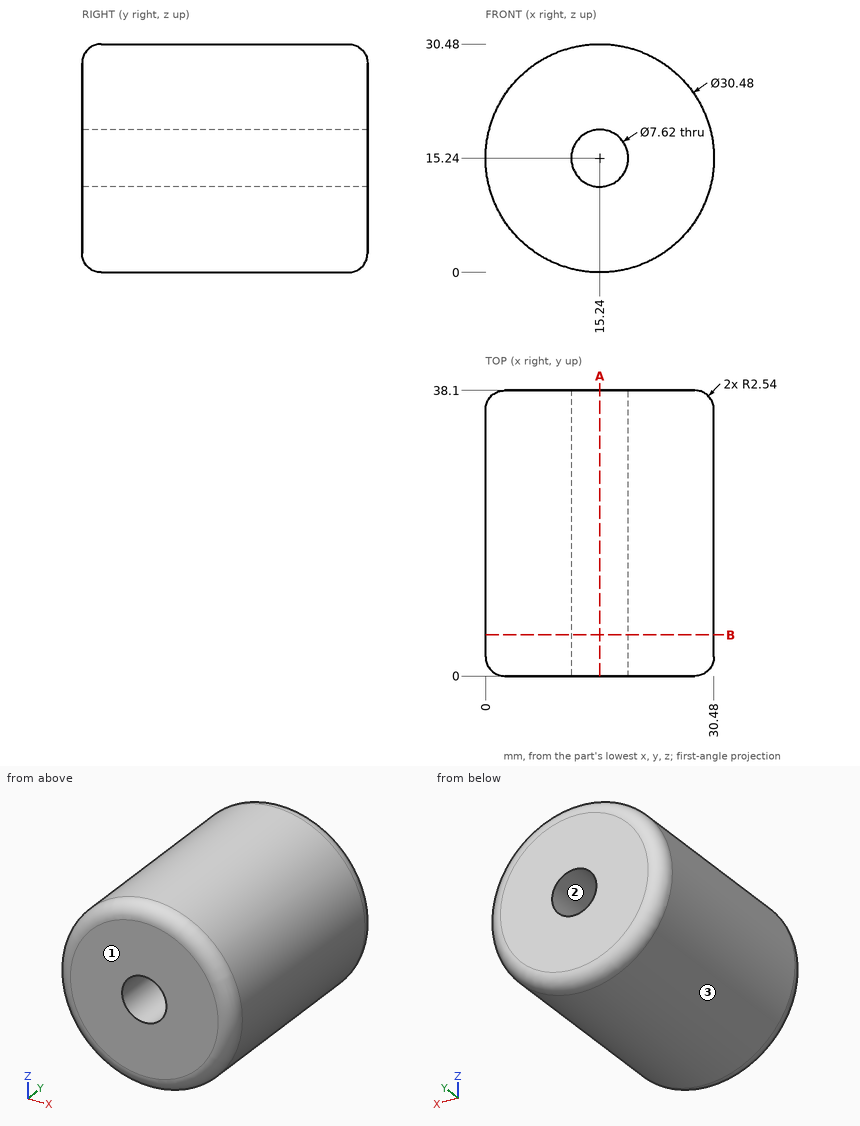
Source: three-view drawing plus pictorial views. Frame: mm from the lowest corner of the part. Give positions to 0.01 mm unless a question says otherwise; leave off trailing zeros. Loops run counter-clockwise (first coordinate to the right, second up) from the corner with the lowest first, then second, coordinate; pieces in that order, holes last. Notation, with made-up numbers: M -16,28 L 19,28 A34 cw 19,61 Z; hole C -27,-28.5 d8. An arc over 180 degrees is marked long. Use CSV: the item, a comma, the result in double quotes.
(1) Section B-B, the plane y = 5.5. Return loops of the section in (x, z).
Outcome:
outline,"C 15.24,15.24 d30.48; hole C 15.24,15.24 d7.62"
(2) Pull-direction query (X, two-part tool) for the marked faces 1, 2 and 3; classes: pulls with the +X half, pulls with the -X half, needs draft (parallel to the pull), parting line crosses it, or undercut.
Outcome:
face 1,"needs draft"
face 2,"undercut"
face 3,"parting line crosses it"
(3) Material intervals for L1, parallel to Z at x = 15, y = 17; L2, parallel to Y at x = 5, z = 23, sorted ascending. Write a range as [from, to].
Outcome:
L1,"z = [0, 11.44], [19.04, 30.48]"
L2,"y = [0, 38.1]"
(4) Pin query (flat end, axial travel): P1, Ø6, axis at y = 17.5, z = 12, coming from the -X side; P2, Ø1.5, axis at y = 29, z = 24.5, coming from the +X side; P3, Ø3, axis at x = 7, y = 27, coming from the +Z side. Return the tip coordinate at first contact, or that it passes through.
Outcome:
P1,"stops at x = 0"
P2,"stops at x = 27.88"
P3,"stops at z = 28.91"
(5) Section A-A, the plane x = 15.24. Return loops of the section in (y, z).
Outcome:
outline,"M 0,2.54 A2.54 ccw 2.54,0 L 35.56,0 A2.54 ccw 38.1,2.54 L 38.1,11.43 L 0,11.43 Z; M 0,19.05 L 38.1,19.05 L 38.1,27.94 A2.54 ccw 35.56,30.48 L 2.54,30.48 A2.54 ccw 0,27.94 Z"
